from build123d import *

# Parameters (mm, degrees)
EXTRUDE_1_DEPTH          = 3
SKETCH_2_W               = 36
SKETCH_2_H               = 3
EXTRUDE_2_DEPTH          = 30
CUT_EXTRUDE_1_DEPTH      = 47.281745862
CUT_EXTRUDE_1_DEPTH_BACK = 47.281745862
FILLET_1_R               = 2
FILLET_2_R               = 2


with BuildPart() as part:
    # 草图1 → 凸台-拉伸1 (new body)
    with BuildSketch(Plane(origin=(0, 0, 0), x_dir=(1, 0, 0), z_dir=(0, 1, 0))):
        Polygon((0, 9.489130435), (-18, 9.489130435), (-18, -20.510869565), (0, -20.510869565), (18, -20.510869565), (18, 9.489130435), align=None)
        with BuildLine():
            Line((-10.5, -0.510869565), (-10.5, -15.510869565))
            ThreePointArc((-10.5, -15.510869565), (-12.5, -17.510869565), (-14.5, -15.510869565))
            Line((-14.5, -15.510869565), (-14.5, -0.510869565))
            ThreePointArc((-14.5, -0.510869565), (-12.5, 1.489130435), (-10.5, -0.510869565))
        make_face(mode=Mode.SUBTRACT)
        with BuildLine():
            Line((14.5, -0.510869565), (14.5, -15.510869565))
            ThreePointArc((14.5, -15.510869565), (12.5, -17.510869565), (10.5, -15.510869565))
            Line((10.5, -15.510869565), (10.5, -0.510869565))
            ThreePointArc((10.5, -0.510869565), (12.5, 1.489130435), (14.5, -0.510869565))
        make_face(mode=Mode.SUBTRACT)
    extrude(amount=EXTRUDE_1_DEPTH)

    # 草图2 → 凸台-拉伸2 (add)
    with BuildSketch(Plane(origin=(0, 3, 0), x_dir=(1, 0, 0), z_dir=(0, 1, 0))):
        with Locations((0, 7.989130435)):
            Rectangle(SKETCH_2_W, SKETCH_2_H)
    extrude(amount=EXTRUDE_2_DEPTH)

    # 草图3 → 切除-拉伸1 (cut, two sides: drawn at the far end of the back side and taken through both)
    with BuildSketch(Plane.XY.offset(-6.489130435).offset(-CUT_EXTRUDE_1_DEPTH_BACK)):
        with BuildLine():
            Line((-8, 28), (-8, 10))
            ThreePointArc((-8, 10), (-10, 8), (-12, 10))
            Line((-12, 10), (-12, 28))
            ThreePointArc((-12, 28), (-10, 30), (-8, 28))
        make_face()
        with BuildLine():
            Line((8, 28), (8, 10))
            ThreePointArc((8, 10), (10, 8), (12, 10))
            Line((12, 10), (12, 28))
            ThreePointArc((12, 28), (10, 30), (8, 28))
        make_face()
    extrude(amount=CUT_EXTRUDE_1_DEPTH + CUT_EXTRUDE_1_DEPTH_BACK, mode=Mode.SUBTRACT)

    # 圆角1
    fillet_1_edges = [part.edges().sort_by_distance(p)[0] for p in [
        (18, 1.5, 20.510869565),
        (-18, 1.5, 20.510869565),
        (-18, 33, -7.989130435),
        (18, 33, -7.989130435),
    ]]
    fillet(fillet_1_edges, radius=FILLET_1_R)

    # 圆角2
    fillet_2_edges = [part.edges().sort_by_distance(p)[0] for p in [
        (0, 3, -6.489130435),
    ]]
    fillet(fillet_2_edges, radius=FILLET_2_R)


solid = part.part
Work out the finished part from the listing and answer in its coordinate system (mm). A direction names the side the tool comes from. Round coordinates to 2 decimals unless told otherwise and drop trailing zeros. Write each loop counter-clockwise with the first axis right and the second up, starting at its lowest first coordinate (ties: lowest second). Pieces come first, ordered by that corner, then holes. Notation, with made-up numbers: (43.5, 80) - (53.5, 80) arc R3 cw to (53.5, 84) - close; hole circle Ø6 at (58, 9). An arc over 180 degrees is marked (long way). Answer in a Markdown table with one row per item. Add a question column.
1. For faces 5 (the cylindrical face through (-12.46, 1.48, 17.51)), 6 (the cylindrical face through (-10, 8, -8)), 7 (the flat face through (0, 1, 20.511)), determine the directions among +Z, -Z, +X, -X, +Y, -Y from which every point of the face is accessible in a straight line to the end or side of a thin tool.
2. A cutting plane is placed at C-C, the plane y = 15. Determine the outline of the cut face in (x, z), and give its area (3 significant figures).
3. A cutting plane is placed at D-D, the plane y = 2.5. Determine the outline of the cut face in (x, z).
4. Given pin 1 (6 mm diameter, centred on x = 0.5, z = 0.5, fed in from +Y); pin 2 (2 mm diameter, centred on x = 7, y = 21.5, fed in from +Z), each flat-ended and moving along its own axis, determine where each tip first touches the part or whether it passes through.
5. A cutting plane is placed at B-B, the plane x = 12.5. Determine the outline of the cut face in (y, z).
6. Find the intervals of material crossed by line 1 along X through (y, z) = (2, 8.75); line 2 along Z through (x, y) = (-3, 19.5); line 3 along X through (y, z) = (9, -7.5), in increasing order. Write a range as from..to.
7. A cutting plane is placed at A-A, the plane z = 3.5. Determine the outline of the cut face in (x, y).
8. The mould has two halves that part along X. Classify faces 1 (the flat face through (-12, 19, -8)), 2 (the flat face through (0, 0, 5)), 3 (the flat face through (-18, 10, -7)), 4 (the cylindrical face through (12.46, 1.48, -1.49)): +X half, -X half, draft (parallel to the pull), parting line (faces both ways), or undercut.
Worked out:
| question | item | result |
|---|---|---|
| 1 | face 5 | +Y, -Y |
| 1 | face 6 | +Z, -Z |
| 1 | face 7 | +Z, +X, -X, +Y, -Y |
| 2 | outline | (-18, -9.49) - (-12, -9.49) - (-12, -6.49) - (-18, -6.49) - close; (-8, -9.49) - (8, -9.49) - (8, -6.49) - (-8, -6.49) - close; (12, -9.49) - (18, -9.49) - (18, -6.49) - (12, -6.49) - close |
| 2 | area | 84.0 mm^2 |
| 3 | outline | (-18, -9.49) - (18, -9.49) - (18, 18.51) arc R2 ccw to (16, 20.51) - (-16, 20.51) arc R2 ccw to (-18, 18.51) - close; hole (-14.5, 0.51) arc R2 ccw to (-10.5, 0.51) - (-10.5, 15.51) arc R2 ccw to (-14.5, 15.51) - close; hole (10.5, 0.51) arc R2 ccw to (14.5, 0.51) - (14.5, 15.51) arc R2 ccw to (10.5, 15.51) - close |
| 4 | pin 1 | y = 3 |
| 4 | pin 2 | z = -6.49 |
| 5 | outline | (0, -9.49) - (33, -9.49) - (33, -6.49) - (5, -6.49) arc R2 cw to (3, -4.49) - (3, -1.49) - (0, -1.49) - close; (0, 17.51) - (3, 17.51) - (3, 20.51) - (0, 20.51) - close |
| 6 | line 1 | -18..-14.5, -10.5..10.5, 14.5..18 |
| 6 | line 2 | -9.49..-6.49 |
| 6 | line 3 | -18..-11.73, -8.27..8.27, 11.73..18 |
| 7 | outline | (-18, 0) - (-14.5, 0) - (-14.5, 3) - (-18, 3) - close; (-10.5, 0) - (10.5, 0) - (10.5, 3) - (-10.5, 3) - close; (14.5, 0) - (18, 0) - (18, 3) - (14.5, 3) - close |
| 8 | face 1 | undercut |
| 8 | face 2 | draft |
| 8 | face 3 | -X half |
| 8 | face 4 | undercut |
